Here's how the part is built. I have some questions about the finished solid (model axes, mm). Round coordinates to 2 decimals unless told otherwise and drop trailing zeros. Loops run counter-clockwise (first coordinate to the right, second up) from the corner with the lowest first, then second, coordinate; pieces in that order, holes last. Notation, with made-up numbers: M 61.25,22.5 L 89.25,22.5 A29 ccw 89.25,53.5 Z; hole C 66.5,-0.5 d3. An arc over 180 degrees is marked long. Use a Markdown table: item, result.
```python
from build123d import *

# Parameters (mm, degrees)
F0_R     = 2.5
F1_DEPTH = 300


with BuildPart() as f1:
    # F0 (on Top) → F1 (new body)
    with BuildSketch(Plane.XY):
        Polygon((-52.643933, -68.08899), (-52.643933, -81.08899), (-39.643933, -81.08899), (-39.643933, -79.08899), (-35.643933, -79.08899), (-35.643933, -81.08899), (-22.643933, -81.08899), (-22.643933, -68.08899), (-24.643933, -68.08899), (-24.643933, -64.08899), (-22.643933, -64.08899), (-22.643933, -51.08899), (-35.643933, -51.08899), (-35.643933, -53.08899), (-39.643933, -53.08899), (-39.643933, -51.08899), (-52.643933, -51.08899), (-52.643933, -64.08899), (-50.643933, -64.08899), (-50.643933, -68.08899), align=None)
        with Locations((-37.643933, -66.08899)):
            Circle(F0_R, mode=Mode.SUBTRACT)
    extrude(amount=F1_DEPTH)


solid = f1.part
```
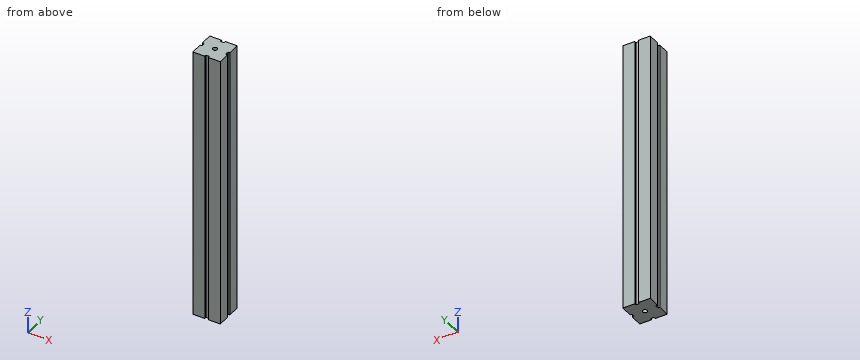
Q1. Imagine slicing it at A-A, the plane z = 80. Please give me the cut outline in (x, y).
Return value:
| item | result |
|---|---|
| outline | M -52.64,-81.09 L -39.64,-81.09 L -39.64,-79.09 L -35.64,-79.09 L -35.64,-81.09 L -22.64,-81.09 L -22.64,-68.09 L -24.64,-68.09 L -24.64,-64.09 L -22.64,-64.09 L -22.64,-51.09 L -35.64,-51.09 L -35.64,-53.09 L -39.64,-53.09 L -39.64,-51.09 L -52.64,-51.09 L -52.64,-64.09 L -50.64,-64.09 L -50.64,-68.09 L -52.64,-68.09 Z; hole C -37.64,-66.09 d5 |
Q2. Will these pins go through, and if not, where does the flat tip stop? P1, Ø1.2, axis at x = -37, z = 148.5, coming from the +Y side; P2, Ø3, axis at y = -66.5, z = 128.5, coming from the -X side; P3, Ø2, axis at x = -38.5, z = 139.5, coming from the -Y side.
Return value:
| item | result |
|---|---|
| P1 | stops at y = -53.09 |
| P2 | stops at x = -50.64 |
| P3 | stops at y = -79.09 |
Q3. I need wall thicknesses on line 1 (X direction, y = -52.75, z = 106); line 2 (Y direction, x = -51, z = 232); line 3 (Y direction, x = -37.75, z = 128). Which ranges of each line are inside material? Lowest first, please. Write a range as from..to.
Return value:
| item | result |
|---|---|
| line 1 | x = -52.64..-39.64, -35.64..-22.64 |
| line 2 | y = -81.09..-68.09, -64.09..-51.09 |
| line 3 | y = -79.09..-68.59, -63.59..-53.09 |
